Autodesk Inventor part; units mm, degrees
ref_plane "YZ Plane" through (0, 0, 0) normal (1, 0, 0) x (0, 1, 0)
ref_plane "XZ Plane" through (0, 0, 0) normal (0, 1, 0) x (-1, 0, 0)
ref_plane "XY Plane" through (0, 0, 0) normal (0, 0, 1) x (1, 0, 0)
sketch "Sketch1" plane through (0, 0, 0) normal (0, 0, 1) x (1, 0, 0)
  line L0 (0, 0) -> (23, 0) construction
  line L1 (23, 0) -> (23, 6) construction
  line L2 (23, 6) -> (0, 6) construction
  line L3 (0, 6) -> (0, 0) construction
  line L4 (0, 3) -> (23, 3) construction
  line L5 (11.5, 0) -> (11.5, 3) construction
  line L6 (11.5, 3) -> (11.5, 6) construction
  line L7 (11.5, 1.5) -> (0, 1.5) construction
  line L8 (11.5, 4.5) -> (23, 4.5) construction
  line L9 (0, 1.5) -> (11.5, 1.5) construction
  line L10 (1.5, 3) -> (10, 3)
  line L11 (10, 0) -> (1.5, 0)
  arc A0 (1.5, 3) -> (1.5, 0) centre (1.5, 1.5) ccw
  arc A1 (10, 0) -> (10, 3) centre (10, 1.5) ccw
  line L12 (11.5, 4.5) -> (23, 4.5) construction
  line L13 (13, 6) -> (21.5, 6)
  line L14 (21.5, 3) -> (13, 3)
  arc A2 (13, 6) -> (13, 3) centre (13, 4.5) ccw
  arc A3 (21.5, 3) -> (21.5, 6) centre (21.5, 4.5) ccw
  line L15 (10, 1.5) -> (13, 4.5) construction
  line L16 (11.0607, 0.4393) -> (14.0607, 3.4393)
  line L17 (11.9393, 5.5607) -> (8.9393, 2.5607)
  arc A4 (8.9393, 2.5607) -> (11.0607, 0.4393) centre (10, 1.5) ccw
  arc A5 (14.0607, 3.4393) -> (11.9393, 5.5607) centre (13, 4.5) ccw
  point P0 (5.75, 1.5)
  point P1 (17.25, 4.5)
  point P2 (11.5, 3)
  point P3 (9.3787, 3)
  point P4 (13.6213, 3)
  dimension "d6" = 23
  dimension "d7" = 6
  dimension "d8" = 3
extrude "Extrusion1" add sketch "Sketch1" along normal blind 308
properties part number "Door Seal" material "Rubber"
The model under review builds one solid part; all positions refer to its coordinate system, in mm. A direction names the side the tool comes from. Give positions to 0.01 mm unless a question says otherwise; leave off trailing zeros. Write each loop counter-clockwise with the first axis right and the second up, starting at its lowest first coordinate (ties: lowest second). Pieces come first, ordered by that corner, then holes. Notation, with made-up numbers: (53, 20) -> (105, 20) arc R9 ccw to (105, 31) -> close; hole circle Ø4 at (89.5, 63.25). An arc over 180 degrees is marked (long way). Answer in a Markdown table with one row per item.
1) Tool access review of faces 1 (the flat face through (18, 3, 152)), 2 (the flat face through (5, 3, 152)), 3 (the flat face through (6, 0, 152)): name each direction out of +Z, -Z, +X, -X, +Y, -Y from which nothing blocks a thin tool from reaching the whole face with its end or side.
Worked answers:
| item | result |
|---|---|
| face 1 | +Z, -Z, +X, -Y |
| face 2 | +Z, -Z, -X, +Y |
| face 3 | +Z, -Z, +X, -X, -Y |
2) Add section B-B on y = 4.5. State the section outline as (x, z) points.
Worked answers:
| item | result |
|---|---|
| outline | (10.88, 0) -> (23, 0) -> (23, 308) -> (10.88, 308) -> close |
3) For L1, parallel to Y at x = 6, z = 24; L2, parallel to Y at x = 20.5, z = 110; L3, parallel to X at y = 3.5, z = 38.5, list the stretches that pass through material, from the lowest coordinate up. Write a range as [from, to].
Worked answers:
| item | result |
|---|---|
| L1 | [0, 3] |
| L2 | [3, 6] |
| L3 | [9.88, 22.62] |
4) Clearance check with flat-ended pins moving along their axes: P1, Ø1.5, axis at y = 1, z = 270, coming from the +X side; P2, Ø2, axis at x = 17, z = 118.5, coming from the -Y side; P3, Ø2.5, axis at x = 6, z = 103, coming from the +Y side. State where each tip first meets the part, or that it passes through.
Worked answers:
| item | result |
|---|---|
| P1 | x = 12.37 |
| P2 | y = 3 |
| P3 | y = 3 |
5) Add section A-A on z = 175.5. State the section outline as (x, y) points.
Worked answers:
| item | result |
|---|---|
| outline | (1.5, 0) -> (10, 0) arc R1.5 ccw to (11.06, 0.44) -> (13.62, 3) -> (21.5, 3) arc R1.5 ccw to (21.5, 6) -> (13, 6) arc R1.5 ccw to (11.94, 5.56) -> (9.38, 3) -> (1.5, 3) arc R1.5 ccw to start |
